from build123d import *

# Parameters (mm, degrees)
ESQUISSE1_R        = 6.1
ESQUISSE1_R_2      = 2.4
BOSS_EXTRU_1_DEPTH = 5
CONG_1_R           = 10
CONG_2_R           = 20


with BuildPart() as part:
    # Esquisse1 → Boss.-Extru.1 (new body)
    with BuildSketch(Plane.XY):
        with BuildLine():
            Line((13.228756555, 15), (377.702263695, 15))
            ThreePointArc((377.702263695, 15), (377.67197868, 15.744094767), (377.640227758, 16.488128424))
            ThreePointArc((377.640227758, 16.488128424), (398.659662111, 39.426815821), (421.598349508, 18.407381468))
            ThreePointArc((421.598349508, 18.407381468), (421.669280552, 16.703827075), (421.733328064, 15))
            Line((421.733328064, 15), (500, 15))
            Line((500, 15), (500, -15))
            Line((500, -15), (421.733328064, -15))
            ThreePointArc((421.733328064, -15), (421.669280552, -16.703827075), (421.598349508, -18.407381468))
            ThreePointArc((421.598349508, -18.407381468), (398.659662111, -39.426815821), (377.640227758, -16.488128424))
            ThreePointArc((377.640227758, -16.488128424), (377.67197868, -15.744094767), (377.702263695, -15))
            Line((377.702263695, -15), (13.228756555, -15))
            ThreePointArc((13.228756555, -15), (-20, 0), (13.228756555, 15))
        make_face()
        Circle(ESQUISSE1_R, mode=Mode.SUBTRACT)
        with Locations((350, 0)):
            Circle(ESQUISSE1_R_2, mode=Mode.SUBTRACT)
        with BuildLine():
            ThreePointArc((392.625951082, -17.142419235), (393, 0), (392.625951082, 17.142419235))
            ThreePointArc((392.625951082, 17.142419235), (399.313952921, 24.441092497), (406.612626184, 17.753090658))
            ThreePointArc((406.612626184, 17.753090658), (407, 0), (406.612626184, -17.753090658))
            ThreePointArc((406.612626184, -17.753090658), (399.313952921, -24.441092497), (392.625951082, -17.142419235))
        make_face(mode=Mode.SUBTRACT)
    extrude(amount=BOSS_EXTRU_1_DEPTH)

    # Congé1
    cong_1_edges = [part.edges().sort_by_distance(p)[0] for p in [
        (13.228756555, 15, 2.5),
        (13.228756555, -15, 2.5),
    ]]
    fillet(cong_1_edges, radius=CONG_1_R)

    # Congé2
    cong_2_edges = [part.edges().sort_by_distance(p)[0] for p in [
        (421.733328064, 15, 2.5),
        (421.733328064, -15, 2.5),
        (377.702263695, 15, 2.5),
        (377.702263695, -15, 2.5),
    ]]
    fillet(cong_2_edges, radius=CONG_2_R)


solid = part.part
For this review, take the finished solid that the model builds, in its own axes (mm). Round coordinates to 2 decimals unless told otherwise and drop trailing zeros. Order: outer loops, then holes, each group sorted by start corner. A loop starts at its lowest first (then second) coordinate and runs counter-clockwise, first axis right, second up. Notation, with made-up numbers: (89, -17) -> (129, -17) arc R30 ccw to (129, 6) -> close; hole circle Ø8 at (49.25, 45.25). An arc over 180 degrees is marked (long way). Write item = value, one per line. Start each with the question number.
1) Take a section at D-D on y = -32. State the section outline as (x, z) points, plus the area to 3 significant figures.
2) Take a section at A-A on x = 0. State the section outline as (y, z) points.
3) To check wall thickness, follow line 1 (Y direction, x = 350, z = 1.3); line 2 (Y direction, x = 0, z = 2); line 3 (X direction, y = 2, z = 2.9). State the ranges of each line that lie inside material, in increasing order. Write a range as from..to.
4) Insertion check: pin 1 (2.5 mm diameter, centred on x = 140, z = 2.5, fed in from +Y); pin 2 (2.5 mm diameter, centred on x = 109, z = 3, fed in from -Y). Each pin has a flat end and moves straight along its axis. Give the tip position at first contact, or say it passes through.
5) The part is to be moulded in two halves that separate along Y. For faces 1 (the face through (-6.094, 0.268, 2.465)), 2 (the face through (-19.99, -0.6, 2.46)), 3 (the face through (244, 1, 5)), say which applies: +Y half, -Y half, draft (parallel to the pull), parting line (faces both ways), or undercut.
6) Take a section at B-B on x = 83.5. State the section outline as (y, z) points.
7) Take a section at C-C on z = 2.5. Count the separate pieces of the cut face and the enclosed holes in it, plus the area to 3 significant figures.
Verdict:
q1.outline = (383.12, 0) -> (416.12, 0) -> (416.12, 5) -> (383.12, 5) -> close
q1.area = 165 mm2
q2.outline = (-20, 0) -> (-6.1, 0) -> (-6.1, 5) -> (-20, 5) -> close; (6.1, 0) -> (20, 0) -> (20, 5) -> (6.1, 5) -> close
q3.line_1 = -15..-2.4, 2.4..15
q3.line_2 = -20..-6.1, 6.1..20
q3.line_3 = -19.9..-5.76, 5.76..348.67, 351.33..392.99, 407..500
q4.pin_1 = 15
q4.pin_2 = -15
q5.face_1 = undercut
q5.face_2 = parting line
q5.face_3 = draft
q6.outline = (-15, 0) -> (15, 0) -> (15, 5) -> (-15, 5) -> close
q7.separate_pieces = 1
q7.enclosed_holes = 3
q7.area = 16,800 mm2
